Geometry check sheet. Reference: the model listing, model coordinates, mm. Face numbers are marked on the shaded views. A direction names the side the tool comes from. Coordinates: 2 decimals unless noted, no trailing zeros. Write each loop counter-clockwise with the first axis right and the second up, starting at its lowest first coordinate (ties: lowest second). Pieces come first, ordered by that corner, then holes. Notation, with made-up numbers: M 64.5,-3.75 L 109.5,-3.75 A36 ccw 109.5,35.25 Z; hole C 48,41.25 d3. An arc over 180 degrees is marked long. Put each result on its own line as item: value. Start each with the question number.
1) Cross-section at D-D on x = 40.75. Record the cut outline in (y, z) (3 decimals).
2) Cross-section at C-C on x = 47.25. Record the cut outline in (y, z).
3) Set-up check for the marked faces 5, 6 and 7: record each of +Z, -Z, +X, -X, +Y, -Y from which the full face is reachable in a straight line by a thin tool's end or side.
4) Cross-section at B-B on z = -8.75. Record the cut outline in (x, y) (3 decimals), plus the area to 3 significant figures.
5) Gauge pin test, flat ends, axial feed: pin 1 (9 mm diameter, centred on y = 19.5, z = 3, fed in from +X); pin 2 (7 mm diameter, centred on y = 23.5, z = 5.5, fed in from -X); pin 3 (3 mm diameter, centred on x = 36.42, y = 33.25, fed in from -Z); pin 4 (8 mm diameter, centred on y = 35.5, z = -5.5, fed in from -X). Record the tip position at first contact, or that the pin passes through.
6) Cross-section at A-A on y = 21.25. Record the cut outline in (x, z) (3 decimals).
7) Mould release check, pull along Z, two halves, no side actions. Record for the marked faces 1, 2, 3 and 4: released by +Z, released by -Z, zero draft, split by the parting line, or undercut.
8) Scan lines: line 1 along X through (y, z) = (19.5, 7.25); line 2 along Y through (x, z) = (41.75, -8.75) (3 decimals); line 3 along Y through (x, z) = (34, 2.5). Record each from-to range of solid material in increasing order.
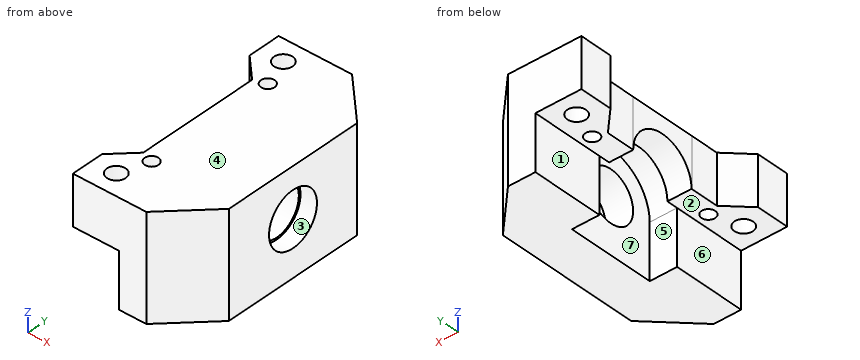
from build123d import *

# Parameters (mm, degrees)
ESQUISSE1_R                               = 1.7
BOSS_EXTRU_1_DEPTH                        = 9
ESQUISSE2_W                               = 13.000000001
ESQUISSE2_H                               = 42.5
BOSS_EXTRU_2_DEPTH                        = 19
ESQUISSE4_R                               = 6.025
ENL_V_MAT_EXTRU_1_DEPTH                   = 4.4
ENL_V_MAT_EXTRU_2_DEPTH                   = 5
ESQUISSE6_R                               = 4.6
ENL_V_MAT_EXTRU_3_DEPTH                   = 9
CHANFREIN1_SIZE                           = 8
TROU_POUR_TARAUDAGE_POUR_TROU_TARAUD_M3_D = 2.5
ESQUISSE9_R                               = 4.95
ENL_V_MAT_EXTRU_4_DEPTH                   = 3


with BuildPart() as part:
    # Esquisse1 → Boss.-Extru.1 (new body)
    with BuildSketch(Plane.XY):
        Polygon((38.615489841, 27.325), (38.615489841, 15.175), (38.61548984, 0), (30.21548984, 0), (30.21548984, 6), (34.21548984, 10), (34.215489841, 15.175), (34.215489841, 27.325), (34.21548984, 32.5), (30.21548984, 36.5), (30.21548984, 42.5), (38.61548984, 42.5), align=None)
        with Locations((34.61548984, 4)):
            Circle(ESQUISSE1_R, mode=Mode.SUBTRACT)
        with Locations((34.61548984, 38.5)):
            Circle(ESQUISSE1_R, mode=Mode.SUBTRACT)
    extrude(amount=BOSS_EXTRU_1_DEPTH)

    # Esquisse2 → Boss.-Extru.2 (add)
    with BuildSketch(Plane.XY.offset(9)):
        with Locations((45.115489841, 21.25)):
            Rectangle(ESQUISSE2_W, ESQUISSE2_H)
    extrude(amount=-BOSS_EXTRU_2_DEPTH)

    # Esquisse4 → Enlèv. mat.-Extru.1 (cut)
    with BuildSketch(Plane.ZY.offset(-34.215489841)):
        with Locations((0, 21.25)):
            Circle(ESQUISSE4_R)
    extrude(amount=-ENL_V_MAT_EXTRU_1_DEPTH, mode=Mode.SUBTRACT)

    # Esquisse5 → Enlèv. mat.-Extru.2 (cut)
    with BuildSketch(Plane.ZY.offset(-38.61548984)):
        with BuildLine():
            Line((0, 29.275), (-10, 29.275))
            Line((-10, 29.275), (-10, 13.225))
            Line((-10, 13.225), (0, 13.225))
            ThreePointArc((0, 13.225), (8.025, 21.25), (0, 29.275))
        make_face()
    extrude(amount=-ENL_V_MAT_EXTRU_2_DEPTH, mode=Mode.SUBTRACT)

    # Esquisse6 → Enlèv. mat.-Extru.3 (cut, through all)
    with BuildSketch(Plane.ZY.offset(-43.61548984)):
        with Locations((0, 21.25)):
            Circle(ESQUISSE6_R)
    extrude(amount=-ENL_V_MAT_EXTRU_3_DEPTH, mode=Mode.SUBTRACT)

    # Chanfrein1
    chanfrein1_edges = [part.edges().sort_by_distance(p)[0] for p in [
        (51.615489841, 0, -0.5),
        (51.615489841, 42.5, -0.5),
    ]]
    chamfer(chanfrein1_edges, length=CHANFREIN1_SIZE)

    # Trou pour taraudage pour trou taraudé M31 (through all)
    with Locations(Plane.XY.offset(9)):
        with Locations((36.41548984, 33.25), (36.41548984, 9.25)):
            Hole(TROU_POUR_TARAUDAGE_POUR_TROU_TARAUD_M3_D / 2)

    # Esquisse9 → Enlèv. mat.-Extru.4 (cut)
    with BuildSketch(Plane(origin=(51.615489841, 0, 0), x_dir=(0, 0, -1), z_dir=(1, 0, 0))):
        with Locations((0, 21.25)):
            Circle(ESQUISSE9_R)
    extrude(amount=-ENL_V_MAT_EXTRU_4_DEPTH, mode=Mode.SUBTRACT)


solid = part.part
Answer key:
1. outline: M 0,-10 L 13.225,-10 L 13.225,0 A8.025 cw 29.275,0 L 29.275,-10 L 42.5,-10 L 42.5,9 L 0,9 Z
2. outline: M 3.63,-10 L 38.87,-10 L 38.87,9 L 3.63,9 Z; hole C 21.25,0 d9.2
3. face 5: -Z, -X
3. face 6: -Z, -X, +Y, -Y
3. face 7: -Z
4. outline: M 38.615,0 L 43.615,0 L 51.615,8 L 51.615,34.5 L 43.615,42.5 L 38.615,42.5 L 38.615,29.275 L 43.615,29.275 L 43.615,13.225 L 38.615,13.225 Z
4. area: 408 mm²
5. pin 1: stops at x = 51.62
5. pin 2: stops at x = 34.22
5. pin 3: stops at z = 0
5. pin 4: stops at x = 38.62
6. outline: M 34.215,6.025 L 38.615,6.025 L 38.615,8.025 L 43.615,8.025 L 43.615,4.6 L 48.615,4.6 L 48.615,4.95 L 51.615,4.95 L 51.615,9 L 34.215,9 Z; M 43.615,-10 L 51.615,-10 L 51.615,-4.95 L 48.615,-4.95 L 48.615,-4.6 L 43.615,-4.6 Z
7. face 1: zero draft
7. face 2: released by -Z
7. face 3: undercut
7. face 4: released by +Z
8. line 1: x = 34.22 to 38.62, 43.62 to 51.62
8. line 2: y = 0 to 13.225, 29.275 to 42.5
8. line 3: y = 0 to 2.42, 5.58 to 9.78, 32.72 to 36.92, 40.08 to 42.5
